CAD build for the part. Positions are in the model's coordinates, mm. A direction names the side the tool comes from. Coordinates: 2 decimals unless noted, no trailing zeros. Order: outer loops, then holes, each group sorted by start corner. A loop starts at its lowest first (then second) coordinate and runs counter-clockwise, first axis right, second up. Notation, with made-up numbers: M -7,-28 L 17,-28 A11 ccw 17,-8 Z; hole C 37.25,-38 d10. An arc over 180 degrees is marked long. One line per item, written item: value.
Autodesk Inventor part; units mm, degrees
ref_plane "YZ Plane" through (0, 0, 0) normal (1, 0, 0) x (0, 1, 0)
ref_plane "XZ Plane" through (0, 0, 0) normal (0, 1, 0) x (-1, 0, 0)
ref_plane "XY Plane" through (0, 0, 0) normal (0, 0, 1) x (1, 0, 0)
sketch "Skizze1" plane through (0, 0, 0) normal (0, 0, 1) x (1, 0, 0)
  line L0 (-8.4, 0) -> (8.4, 0)
  line L1 (0, -3.5) -> (0, 3.5)
  line L2 (-6, 2.5) -> (6, 2.5)
  line L3 (6, 2.5) -> (6, -2.5)
  line L4 (6, -2.5) -> (-6, -2.5)
  line L5 (-6, -2.5) -> (-6, 2.5)
  point P0 (0, 0)
  dimension "d0" = 12
  dimension "d1" = 5
extrude "Extrusion1" add sketch "Skizze1" along normal blind 28
sketch "Skizze2" plane through (-6, 2.5, 0) normal (0, 1, 0) x (1, 0, 0)
  line L0 (0, -28) -> (1.5, -28)
  line L1 (1.5, -28) -> (1.5, -20)
  line L2 (1.5, -20) -> (0, -20)
  line L3 (0, -20) -> (0, -28)
  line L4 (12, -28) -> (10.5, -28)
  line L5 (10.5, -28) -> (10.5, -20)
  line L6 (10.5, -20) -> (12, -20)
  line L7 (12, -20) -> (12, -28)
  line L8 (-2.4, 0) -> (14.4, 0)
  line L9 (6, 5.6) -> (6, -33.6)
  point P0 (6, 0)
  dimension "d4" = 9
  dimension "d5" = 8
extrude "Extrusion2" cut sketch "Skizze2" against normal through all
sketch "Skizze3" plane through (0, 0, 0) normal (0, 0, -1) x (-1, 0, 0)
  line L0 (6, 2.5) -> (-6, 2.5)
  line L1 (-2.5, 2.5) -> (2.5, 2.5)
  line L2 (2.5, 2.5) -> (2.5, -1.5)
  line L3 (2.5, -1.5) -> (-2.5, -1.5)
  line L4 (-2.5, -1.5) -> (-2.5, 2.5)
  line L5 (8.4, 0) -> (-8.4, 0)
  line L6 (0, -3.5) -> (0, 3.5)
  point P0 (0, 0)
  dimension "d8" = 5
  dimension "d9" = 4
extrude "Extrusion3" add sketch "Skizze3" along normal blind 10
sketch "Skizze5" plane through (0, 0, 28) normal (0, 0, 1) x (1, 0, 0)
  line L0 (-4.5, 2.5) -> (-4.5, -2.5)
  line L1 (-4.5, -2.5) -> (4.5, -2.5)
  line L2 (4.5, -2.5) -> (4.5, 2.5)
  line L3 (4.5, 2.5) -> (-4.5, 2.5)
  line L4 (-4.5, 0) -> (4.5, 0)
  line L5 (0, 2.5) -> (0, -2.5)
  point P0 (0, 0)
  point P1 (0, 0)
hole "Bohrung2" at (0, 0, 28) direction (0, 0, -1) diameter 1.567 depth 6 tip angle 118
sketch "Skizze6" plane through (2.5, -1.5, 0) normal (1, 0, 0) x (0, 0, -1)
  line L0 (0, 0) -> (0, 4)
  line L1 (10, 4) -> (10, 0)
  line L2 (10, 2) -> (0, 2)
  point P0 (0, 1.5)
  point P1 (8, 2)
  dimension "d28" = 2
hole "Bohrung3" at (2.5, 0.5, -8) direction (-1, 0, 0) diameter 2 end through all countersink diameter 3 countersink angle 90
sketch "Skizze7" plane through (2.5, -1.5, 0) normal (1, 0, 0) x (0, 0, -1)
  circle A0 centre (8, 2) radius 1.5
  line L0 (0, 0) -> (0, 4)
  line L1 (0, 0) -> (10, 0)
  line L2 (10, 4) -> (10, 0)
  line L3 (2, 2) -> (8, 2) construction
  line L4 (2, 3) -> (8, 3)
  line L5 (8, 1) -> (2, 1)
  arc A1 (2, 3) -> (2, 1) centre (2, 2) ccw
  arc A2 (8, 1) -> (8, 3) centre (8, 2) ccw
  point P0 (0, 1.5)
  point P1 (5, 2)
  dimension "d36" = 2
  dimension "d37" = 2
  dimension "d38" = 2
extrude "Extrusion4" cut sketch "Skizze7" against normal through all contours L4 A2 L5 A0 | A0 L5 A1 L4 picked at (7.5, 2)
sketch "Skizze8" plane through (-2.5, -1.5, 0) normal (0, -1, 0) x (1, 0, 0)
  line L0 (5, 0) -> (5, -10)
  line L1 (0, 0) -> (5, 0)
  line L2 (5, 0) -> (5, -4)
  line L3 (5, -4) -> (0, -4)
  line L4 (0, -4) -> (0, 0)
  point P0 (2.5, 0)
  dimension "d41" = 4
extrude "Extrusion5" add sketch "Skizze8" along normal blind 1
sketch "Skizze9" plane through (-2.5, -2.5, 0) normal (-1, 0, 0) x (0, 0, 1)
  arc A0 (-8, 4) -> (-8, 2) centre (-8, 3) ccw
  point P0 (0, 2.5)
hole "Bohrung4" at (-2.5, 0.5, -8) direction (1, 0, 0) diameter 2 end through all countersink diameter 3 countersink angle 90
fillet "Rundung1" radius 2 2 edges at (0, -1.5, -10) (0, 2.5, -10)
sketch "Skizze11" plane through (6, -2.5, 0) normal (1, 0, 0) x (0, 0, -1)
  line L0 (-20, 5) -> (-20, 0)
  line L1 (0, 0) -> (-20, 0)
  line L2 (0, 5) -> (0, 0)
  line L3 (-15, 2.5) -> (-5, 2.5) construction
  line L4 (-15, 4) -> (-5, 4)
  line L5 (-5, 1) -> (-15, 1)
  arc A0 (-15, 4) -> (-15, 1) centre (-15, 2.5) ccw
  arc A1 (-5, 1) -> (-5, 4) centre (-5, 2.5) ccw
  point P0 (0, 2.5)
  point P1 (-10, 2.5)
  dimension "d61" = 3
  dimension "d62" = 2.5
  dimension "d63" = 5
  dimension "d64" = 5
extrude "Extrusion6" cut sketch "Skizze11" against normal through all
sketch "Skizze12" plane through (-4.5, -2.5, 28) normal (0, -1, 0) x (1, 0, 0)
  line L0 (-1.5, -28) -> (-1.5, -8)
  line L1 (2, -28) -> (-1.5, -28)
  line L2 (10.5, -28) -> (10.5, -8)
  line L3 (10.5, -8) -> (9, -8)
  line L4 (4.5, -13) -> (4.5, -23) construction
  line L5 (0.5, -13) -> (0.5, -23)
  line L6 (8.5, -23) -> (8.5, -13)
  arc A0 (8.5, -13) -> (0.5, -13) centre (4.5, -13) ccw
  arc A1 (0.5, -23) -> (8.5, -23) centre (4.5, -23) ccw
  point P0 (4.5, -28)
  point P1 (4.5, -18)
  dimension "d67" = 6
  dimension "d68" = 8
  dimension "d69" = 5
  dimension "d70" = 5
extrude "Extrusion7" cut sketch "Skizze12" against normal through all
properties part number "13_1087_004" material "Titan"
Q1. Slice it at C-C (z = 7). List the corners of the cut face in (x, y).
Recorded:
outline: M -6,-2.5 L -4,-2.5 L -4,-1.5 L -6,-1.5 Z; M -6,1.5 L -4,1.5 L -4,2.5 L -6,2.5 Z; M 4,-2.5 L 6,-2.5 L 6,-1.5 L 4,-1.5 Z; M 4,1.5 L 6,1.5 L 6,2.5 L 4,2.5 Z
Q2. Which spindle directions (+Z, -Z, +X, -X, +Y, -Y) get a long thin tool onto all of the face, cutting with end or side? Do faces 4 (the face through (4, 0, 0)), 5 (the face through (4.5, 0, 24)), 6 (the face through (0, -1.5, -6)), 7 (the face through (-5, -1.5, 10)). Say none if no direction does.
Recorded:
face 4: -Z, +X, +Y, -Y
face 5: +Z, +X, +Y, -Y
face 6: -Z, +X, -X, -Y
face 7: +X, -X
Q3. Slice it at B-B (x = -1.5). Give the number of separate pieces and of enclosed holes in the cut face, plus the area to 3 significant figures.
Recorded:
separate pieces: 2
enclosed holes: 1
area: 80.1 mm^2
Q4. Mould opens along Y. For faces 1 (the face through (-4.1, -2.5, 15.8)), 2 (the face through (0, -0.5, -5)), 3 (the face through (-4.5, 0, 24)) say: released by +Y, released by -Y, zero draft, split by the parting line, or undercut.
Recorded:
face 1: released by -Y
face 2: undercut
face 3: zero draft
Q5. Pin check, flat tip, straight feed: pin 1 Ø0.5 at (x, y) = (1, -2) entering from -Z. Stop position of the tip, or through.
Recorded:
pin 1: stops at z = -4
Q6. Slice it at A-A (z = -3). List the corners of the cut face in (x, y), plus the area to 3 significant figures.
Recorded:
outline: M -2.5,-2.5 L 2.5,-2.5 L 2.5,-0.5 L -2.5,-0.5 Z; M -2.5,1.5 L 2.5,1.5 L 2.5,2.5 L -2.5,2.5 Z
area: 15.0 mm^2
Q7. Drill centre lines: line 1 along X through (y, z) = (1.7, 9.5); line 2 along X through (y, z) = (0, 25.8); line 3 along Y through (x, z) = (0, -4.5). Where is each one in solid material? Low to high.
Recorded:
line 1: x = -6 to -4, 4 to 6
line 2: x = -4.5 to -0.78, 0.78 to 4.5
line 3: y = -1.5 to -0.5, 1.5 to 2.5
